Check sheet for the modelled part. Datum: model origin and axes. Units: mm. A direction names the side the tool comes from. Round coordinates to 2 decimals unless told otherwise and drop trailing zeros. Write each loop counter-clockwise with the first axis right and the second up, starting at its lowest first coordinate (ties: lowest second). Pieces come first, ordered by that corner, then holes.
Item 1: Go/stop test with flat-tipped pins: pin 1 Ø10 at (y, z) = (-23.5, -8.5) entering from -X; pin 2 Ø4 at (x, y) = (25.5, -39) entering from -Z; pin 3 Ø17 at (y, z) = (-25.22, 25.4) entering from -X; pin 4 Ø6.5 at (y, z) = (-21.5, -4.5) entering from +X. Record where each tip stops, or that it passes through.
Item 2: Material ranges on line 1 (Y direction, x = 18, z = 25); line 2 (Z direction, x = 47.5, y = -50); line 3 (Y direction, x = 32, z = 23), recorded low to high.
Item 3: Cross-section at A-A on y = -30.5. Enter the section's corners in (x, z).
Item 4: Cross-section at B-B on z = 29.5. Enter the section's corners in (x, y).
Item 5: Tool access check on faces 5 (the flat face through (24, -9.353, -6)), 6 (the flat face through (19, -50.8, 37)), 7 (the flat face through (11.053, -22, -6)), 8 (the flat face through (24, -34.753, -6)). Record the directions out of +Z, -Z, +X, -X, +Y, -Y that give a thin tool (end or side, any length) a straight path to the whole face; none if there is none.
Item 6: Cross-section at C-C on x = 10. Enter the section's corners in (y, z).
Item 7: Release check for a two-part mould opening along Z. For faces 1 (the cylindrical face through (12.495, -57.061, 26.029)), 2 (the flat face through (24, -22, -12.7)), 3 (the flat face through (36.453, -22, -6)), 4 (the cylindrical face through (25.76, -18.74, 12.94)) record: +Z half, -Z half, draft (parallel to the pull), parting line (faces both ways), or undercut.
Item 8: Cross-section at D-D on x = 28. Enter the section's corners in (y, z).
from build123d import *

# Parameters (mm, degrees)
F0_W     = 50.8
F0_H     = 50.8
F1_DEPTH = 50.8
F2_R     = 12.7
F3_DEPTH = 12.7
F4_R     = 14.045612
F5_DEPTH = 50.8
F6_W     = 25.4
F6_H     = 25.4
F7_DEPTH = 12.7


with BuildPart() as f1:
    # F0 (on Front) → F1 (new body)
    with BuildSketch(Plane.XZ):
        with Locations((25.4, 25.4)):
            Rectangle(F0_W, F0_H)
    extrude(amount=F1_DEPTH)

    # F2 (on face) → F3 (join)
    with BuildSketch(Plane.XZ.offset(50.8)):
        with Locations((25.183003, 25.47081)):
            Circle(F2_R)
    extrude(amount=F3_DEPTH)

    # F4 (on face) → F5 (cut)
    with BuildSketch(Plane.YZ.offset(50.8)):
        with Locations((-25.221433, 25.4)):
            Circle(F4_R)
    extrude(amount=-F5_DEPTH, mode=Mode.SUBTRACT)

    # F6 (on face) → F7 (join)
    with BuildSketch(Plane(origin=(0, 0, 0), x_dir=(1, 0, 0), z_dir=(0, 0, -1))):
        with Locations((23.752804, 22.052956)):
            Rectangle(F6_W, F6_H)
    extrude(amount=F7_DEPTH)


solid = f1.part
Response values:
1. pin 1: stops at x = 11.05
1. pin 2: stops at z = 0
1. pin 3: passes through
1. pin 4: stops at x = 36.45
2. line 1: y = -63.5 to -39.26, -11.18 to 0
2. line 2: z = 0 to 50.8
2. line 3: y = -63.5 to -39.06, -11.38 to 0
3. outline: (0, 0) - (11.05, 0) - (11.05, -12.7) - (36.45, -12.7) - (36.45, 0) - (50.8, 0) - (50.8, 12.38) - (0, 12.38) - close; (0, 38.42) - (50.8, 38.42) - (50.8, 50.8) - (0, 50.8) - close
4. outline: (0, -50.8) - (13.14, -50.8) - (13.14, -63.5) - (37.23, -63.5) - (37.23, -50.8) - (50.8, -50.8) - (50.8, -38.66) - (0, -38.66) - close; (0, -11.79) - (50.8, -11.79) - (50.8, 0) - (0, 0) - close
5. face 5: -Z, +X, -X, +Y
5. face 6: -Y
5. face 7: -Z, -X, +Y, -Y
5. face 8: -Z, +X, -X, -Y
6. outline: (-50.8, 0) - (0, 0) - (0, 50.8) - (-50.8, 50.8) - close; hole circle Ø28.09 at (-25.22, 25.4)
7. face 1: parting line
7. face 2: -Z half
7. face 3: draft
7. face 4: undercut
8. outline: (-63.5, 13.09) - (-50.8, 13.09) - (-50.8, 0) - (-34.75, 0) - (-34.75, -12.7) - (-9.35, -12.7) - (-9.35, 0) - (0, 0) - (0, 50.8) - (-50.8, 50.8) - (-50.8, 37.85) - (-63.5, 37.85) - close; hole circle Ø28.09 at (-25.22, 25.4)
